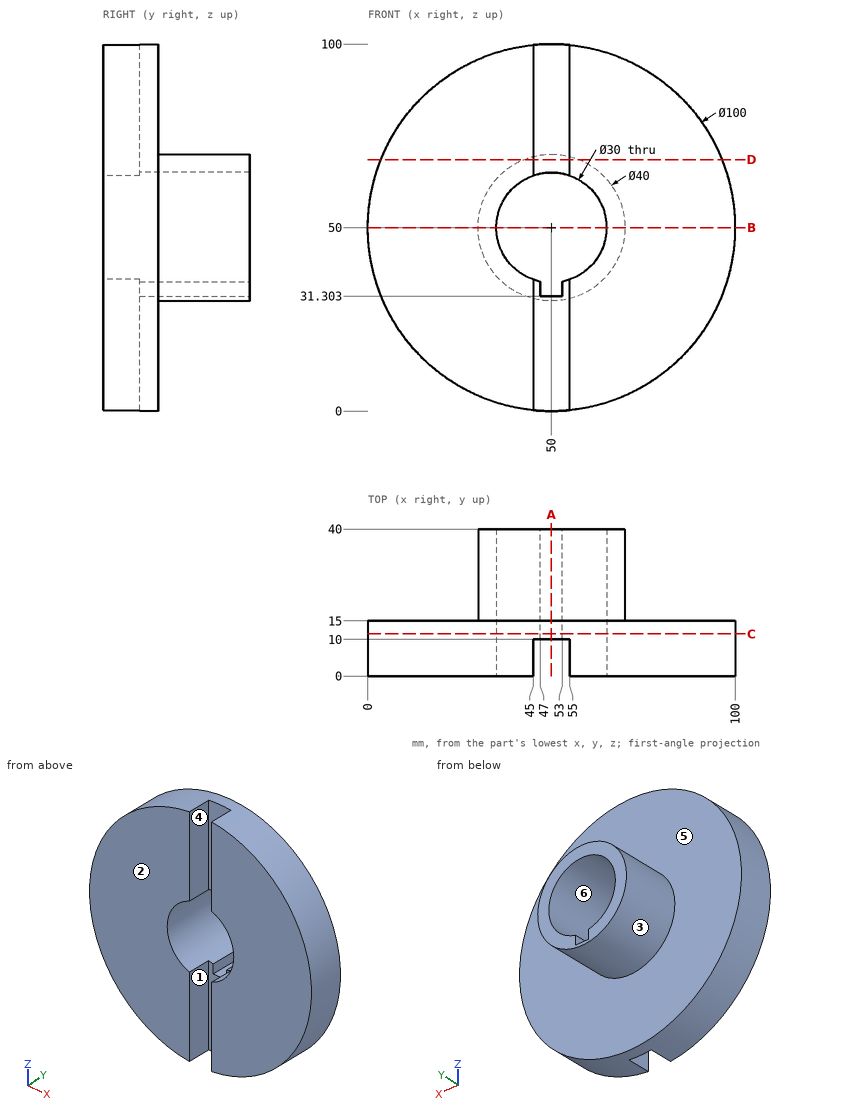
Print and shaded views of the part. All mm, measured from the part's lowest x, y and z. A direction names the side the tool comes from. Round coordinates to 2 decimals unless told otherwise and drop trailing zeros. Write each loop counter-clockwise with the first axis right and the second up, starting at its lowest first coordinate (ties: lowest second). Pieces come first, ordered by that corner, then holes. Notation, with made-up numbers: M 47.25,-2.5 L 88.25,-2.5 A18 cw 88.25,31.5 Z; hole C 78,27 d9. An arc over 180 degrees is marked long. Use a Markdown table: item, result. Add a question column.
1. Slice it at A-A on x = 50. Give the cut face in (y, z).
2. Slice it at D-D on z = 68.5. Give the cut face in (x, y).
3. Pull direction X, two halves, no side cores. Call the marked faces 1, 2, 3 and 4: released by +X, released by -X, zero draft, split by the parting line, or undercut.
4. Flat gauge pins, fed straight in: P1, Ø5, axis at y = 3, z = 11, coming from the -X side; P2, Ø10, axis at y = 9, z = 27, coming from the +X side; P3, Ø5, axis at x = 49.5, y = 28.5, coming from the +Z side. Where does each tip first touch, or does it go through?
5. 3-axis set-ups, long thin cutter, end or side, ignore diameter. For the marked faces 5 and 6: which of +Z, -Z, +X, -X, +Y, -Y reach the whole face in a straight line?
6. Slice it at B-B on z = 50. Give the cut face in (x, y), then the cut area to 3 significant figures.
7. Slice it at C-C on y = 11.5. Give the cut face in (x, z), then the cut area to 3 significant figures.
8. Drill centre lines: probe 1 along X at (y, z) = (19, 50); probe 2 along Z at (x, y) = (50, 12.5); probe 3 along Y at (x, z) = (58.5, 31). Where is each one in solid material? Low to high.
Reply:
| question | item | result |
|---|---|---|
| 1 | outline | M 10,0 L 15,0 L 15,30 L 40,30 L 40,31.3 L 10,31.3 Z; M 10,65 L 40,65 L 40,70 L 15,70 L 15,100 L 10,100 Z |
| 2 | outline | M 3.55,0 L 45,0 L 45,10 L 55,10 L 55,0 L 96.45,0 L 96.45,15 L 57.6,15 L 57.6,40 L 42.4,40 L 42.4,15 L 3.55,15 Z |
| 3 | face 1 | undercut |
| 3 | face 2 | zero draft |
| 3 | face 3 | split by the parting line |
| 3 | face 4 | undercut |
| 4 | P1 | stops at x = 15.83 |
| 4 | P2 | stops at x = 96.65 |
| 4 | P3 | stops at z = 70 |
| 5 | face 5 | +Y |
| 5 | face 6 | +Y, -Y |
| 6 | outline | M 0,0 L 35,0 L 35,40 L 30,40 L 30,15 L 0,15 Z; M 65,0 L 100,0 L 100,15 L 70,15 L 70,40 L 65,40 Z |
| 6 | area | 1,300 mm^2 |
| 7 | outline | C 50,50 d100; hole M 47,31.3 L 53,31.3 L 53,35.3 A15 ccw long 47,35.3 Z |
| 7 | area | 7,120 mm^2 |
| 8 | probe 1 | x = 30 to 35, 65 to 70 |
| 8 | probe 2 | z = 0 to 31.3, 65 to 100 |
| 8 | probe 3 | y = 0 to 15 |
